Autodesk Inventor part; units mm, degrees
ref_plane "YZ Plane" through (0, 0, 0) normal (1, 0, 0) x (0, 1, 0)
ref_plane "XZ Plane" through (0, 0, 0) normal (0, 1, 0) x (-1, 0, 0)
ref_plane "XY Plane" through (0, 0, 0) normal (0, 0, 1) x (1, 0, 0)
sketch "スケッチ1" plane through (0, 0, 0) normal (0, 0, 1) x (1, 0, 0)
  line L0 (35.3, 43.5) -> (-35.3, 43.5)
  line L1 (-35.3, 43.5) -> (-35.3, -43.5)
  line L2 (-35.3, -43.5) -> (35.3, -43.5)
  line L3 (35.3, 43.5) -> (-35.3, -43.5) construction
  line L4 (-35.3, 43.5) -> (35.3, -43.5) construction
  circle A0 centre (-31.3, -39.5) radius 1.6
  circle A1 centre (10.7, -39.5) radius 1.6
  line L5 (29.7, 0) -> (-35.3, 0) construction
  circle A2 centre (-31.3, 39.5) radius 1.6
  circle A3 centre (10.7, 39.5) radius 1.6
  line L6 (14.65, 36.45) -> (-35.1, 36.45)
  line L7 (-35.1, 36.45) -> (-35.1, -36.45)
  line L8 (-35.1, -36.45) -> (14.65, -36.45)
  line L9 (14.65, -36.45) -> (14.65, 36.45)
  line L10 (14.65, 36.45) -> (-35.1, -36.45) construction
  line L11 (-35.1, 36.45) -> (14.65, -36.45) construction
  line L12 (35.3, -24) -> (29.7, -24)
  line L13 (29.7, -24) -> (29.7, 24)
  line L14 (29.7, 24) -> (35.3, 24)
  line L15 (35.3, -43.5) -> (35.3, -24)
  line L16 (35.3, 24) -> (35.3, 43.5)
  line L17 (4.4, 28.9) -> (-34.6, 28.9)
  line L18 (-34.6, 28.9) -> (-34.6, -28.9)
  line L19 (-34.6, -28.9) -> (4.4, -28.9)
  line L20 (4.4, -28.9) -> (4.4, 28.9)
  line L21 (4.4, 28.9) -> (-34.6, -28.9) construction
  line L22 (-34.6, 28.9) -> (4.4, -28.9) construction
  line L23 (-35.3, 11.2) -> (-12.8, 11.2)
  line L24 (-12.8, 11.2) -> (-12.8, 28)
  line L25 (-12.8, 28) -> (-35.3, 28)
  line L26 (-35.3, 11.2) -> (-37.8, 11.2)
  line L27 (-37.8, 11.2) -> (-37.8, 28)
  line L28 (-37.8, 28) -> (-35.3, 28)
  line L29 (-36.3, 7.17) -> (-19.3, 7.17)
  line L30 (-19.3, 7.17) -> (-19.3, -5.93)
  line L31 (-19.3, -5.93) -> (-36.3, -5.93)
  line L32 (-36.3, -5.93) -> (-36.3, 7.17)
  line L33 (-36.3, -12.41) -> (-25.3, -12.41)
  line L34 (-25.3, -12.41) -> (-25.3, -28.01)
  line L35 (-25.3, -28.01) -> (-36.3, -28.01)
  line L36 (-36.3, -28.01) -> (-36.3, -12.41)
  point P0 (0, 0)
  point P1 (-10.225, 0)
  point P2 (-10.225, 0)
  point P3 (-15.1, 0)
  dimension "d0" = 70.6
  dimension "d1" = 87
  dimension "d2" = 3.2
  dimension "d3" = 3.2
  dimension "d4" = 4
  dimension "d5" = 46
  dimension "d6" = 4
  dimension "d7" = 4
  dimension "d8" = 49.75
  dimension "d9" = 72.9
  dimension "d10" = 0.2
  dimension "d11" = 19.5
  dimension "d12" = 5.6
  dimension "d13" = 39
  dimension "d14" = 57.8
  dimension "d15" = 7.55
  dimension "d16" = 0.5
  dimension "d23" = 22.5
  dimension "d24" = 16.8
  dimension "d26" = 2.5
  dimension "d27" = 13.1
  dimension "d28" = 16
  dimension "d29" = 1
  dimension "d37" = 11
  dimension "d38" = 15.6
  dimension "d42" = 15.5
  dimension "d43" = 4.03
  dimension "d44" = 6.48
extrude "押し出し1" add sketch "スケッチ1" along normal blind 1.6 contours L16 L14 L13 L12 L15 L2 L1 L35 L7 L8 L9 L6 L25 L0 | L25 L7 L23 L1 | L23 L7 L29 L1 | L25 L18 L23 L7 | L7 L6 L9 L8 L35 L18 L19 L20 L17 L25 | L29 L7 L31 L1 | L23 L18 L29 L7 | L25 L24 L23 L18 | L18 L17 L20 L19 L35 L34 L33 L31 L30 L29 L23 L24 L25 | L31 L7 L33 L1 | L29 L18 L31 L7 | L33 L7 L35 L1 | L31 L18 L33 L7 | L29 L30 L31 L18 | L33 L18 L35 L7 | L33 L34 L35 L18
extrude "押し出し2" add sketch "スケッチ1" along normal blind 11.79 contours L25 L18 L23 L7 | L7 L6 L9 L8 L35 L18 L19 L20 L17 L25 | L23 L18 L29 L7 | L25 L24 L23 L18 | L18 L17 L20 L19 L35 L34 L33 L31 L30 L29 L23 L24 L25 | L29 L18 L31 L7 | L31 L18 L33 L7 | L29 L30 L31 L18 | L33 L18 L35 L7 | L33 L34 L35 L18
extrude "押し出し3" add sketch "スケッチ1" along normal blind 29.79 contours L25 L24 L23 L18 | L18 L17 L20 L19 L35 L34 L33 L31 L30 L29 L23 L24 L25 | L29 L30 L31 L18 | L33 L34 L35 L18
extrude "押し出し4" add sketch "スケッチ1" against normal blind 14.5 contours L25 L7 L23 L1 | L1 L26 L27 L28 | L25 L18 L23 L7 | L25 L24 L23 L18
extrude "押し出し5" add sketch "スケッチ1" against normal blind 16 contours L29 L7 L31 L1 | L1 L31 L32 L29 | L29 L18 L31 L7 | L29 L30 L31 L18
extrude "押し出し6" add sketch "スケッチ1" against normal blind 6.2 contours L33 L7 L35 L1 | L1 L35 L36 L33 | L33 L18 L35 L7 | L33 L34 L35 L18
equation "\"d7\" = d6"
properties part number "JetsonXavierNX_and_EN715"
The model under review builds one solid part; all positions refer to its coordinate system, in mm. A direction names the side the tool comes from. Coordinates: 2 decimals unless noted, no trailing zeros. Write each loop counter-clockwise with the first axis right and the second up, starting at its lowest first coordinate (ties: lowest second). Pieces come first, ordered by that corner, then holes.
1) Machinability: for faces 4 (the face through (-31, -12.41, -3)), 5 (the face through (-25.3, -20, -3)), 6 (the face through (-12.8, 19, -7)), 7 (the face through (-11, -36.45, 7)), which of the approach directions +Z, -Z, +X, -X, +Y, -Y give a long, thin tool a straight path to every point of the face, cutting with its end or side? Answer none if there is none.
2) The part is to be moulded in two halves that separate along X. For faces 1 (the face through (11.44, -38.08, 0.79)), 2 (the face through (-35.1, 1, 7)), 3 (the face through (4.4, 0, 21)), say which applies: pulls with the +X half, pulls with the -X half, needs draft (parallel to the pull), parting line crosses it, or undercut.
3) Clearance check with flat-ended pins moving along their axes: pin 1 Ø2 at (x, z) = (-29, 23) entering from +Y; pin 2 Ø1.8 at (y, z) = (-9.5, 0.5) entering from +X; pin 3 Ø12 at (x, y) = (-2.5, -5) entering from -Z; pin 4 Ø2.5 at (x, y) = (-31.3, 39.5) entering from -Z. State where each tip first meets the part, or that it passes through.
4) To check wall thickness, follow probe 1 along Y at (x, z) = (-31.3, 0.9); probe 2 along X at (y, z) = (39, 1); probe 3 along Z at (x, y) = (-14, 26). State the ranges of each line that lie inside material, in increasing order.
5) We need section C-C on z = -9.5. State the section outline as (x, y) points.
6) We need section D-D on x = -21. State the section outline as (y, z) points.
7) We need section A-A on y = -39.5. State the section outline as (x, z) points.
8) We need section B-B on x = -31.3. Count the separate pieces of the cut face and the enclosed holes in it, then the cut area to 3 significant figures.
Answer list:
1. face 4: -Z, +X, -X
1. face 5: -Z, +X, -Y
1. face 6: -Z, +X, +Y, -Y
1. face 7: +Z, +X, -X, -Y
2. face 1: undercut
2. face 2: pulls with the -X half
2. face 3: pulls with the +X half
3. pin 1: stops at y = 28.9
3. pin 2: stops at x = 29.7
3. pin 3: stops at z = 0
3. pin 4: passes through
4. probe 1: y = -43.5 to -41.1, -37.9 to 37.9, 41.1 to 43.5
4. probe 2: x = -35.3 to -32.82, -29.78 to 9.18, 12.22 to 35.3
4. probe 3: z = -14.5 to 29.79
5. outline: (-37.8, 11.2) - (-12.8, 11.2) - (-12.8, 28) - (-37.8, 28) - close; (-36.3, -5.93) - (-19.3, -5.93) - (-19.3, 7.17) - (-36.3, 7.17) - close
6. outline: (-43.5, 0) - (-5.93, 0) - (-5.93, -16) - (7.17, -16) - (7.17, 0) - (11.2, 0) - (11.2, -14.5) - (28, -14.5) - (28, 0) - (43.5, 0) - (43.5, 1.6) - (36.45, 1.6) - (36.45, 11.79) - (28.9, 11.79) - (28.9, 29.79) - (-28.9, 29.79) - (-28.9, 11.79) - (-36.45, 11.79) - (-36.45, 1.6) - (-43.5, 1.6) - close
7. outline: (-35.3, 0) - (-32.9, 0) - (-32.9, 1.6) - (-35.3, 1.6) - close; (-29.7, 0) - (9.1, 0) - (9.1, 1.6) - (-29.7, 1.6) - close; (12.3, 0) - (35.3, 0) - (35.3, 1.6) - (12.3, 1.6) - close
8. separate pieces: 3
8. enclosed holes: 0
8. area: 2,460 mm2
